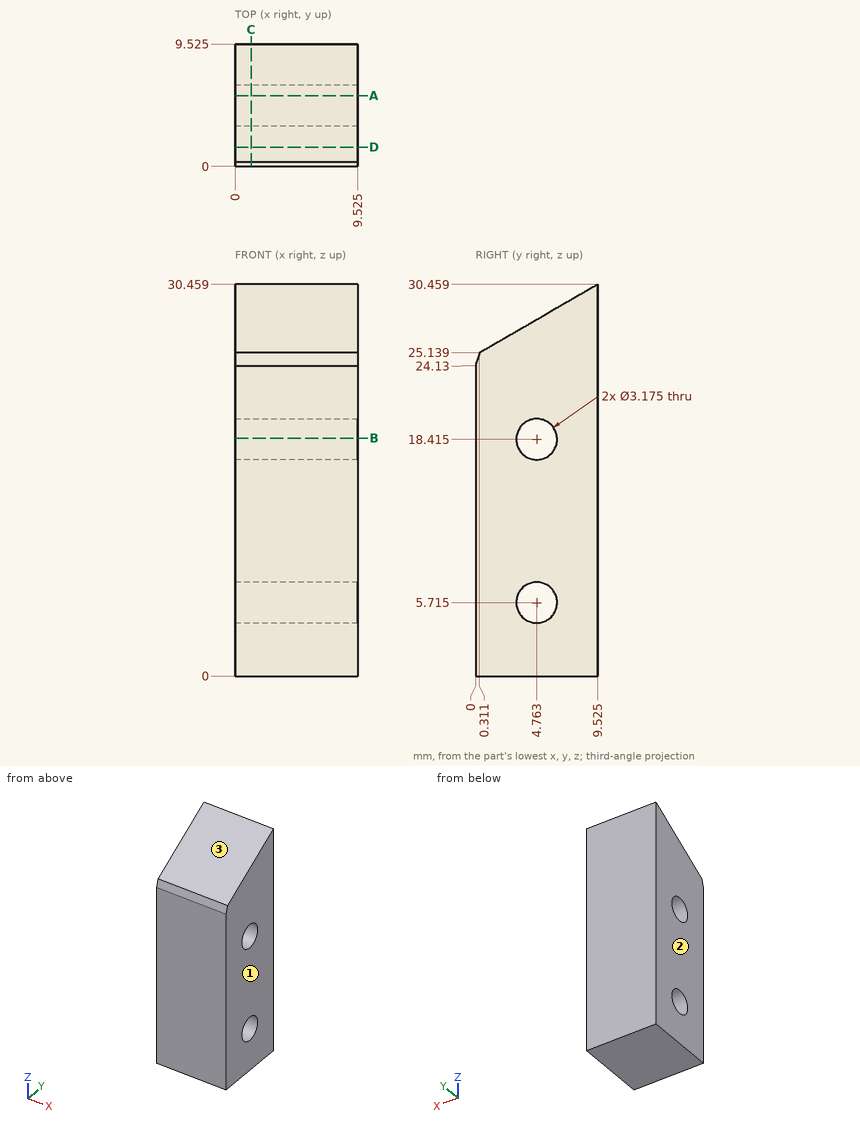
Here's the drawing with two shaded views (mm, measured from the low corner). I have some questions. Round coordinates to 2 decimals unless told otherwise and drop trailing zeros. Order: outer loops, then holes, each group sorted by start corner. A loop starts at its lowest first (then second) coordinate and runs counter-clockwise, first axis right, second up. Notation, with made-up numbers: (71, 12.5) -> (92, 12.5) arc R15 cw to (92, 37.5) -> close; hole circle Ø6 at (3.5, -25.75). An arc over 180 degrees is marked (long way). Write each question's results on one line, items separated by ' | '. Start each with the question number.
Item 1: If we section it at B-B, the plane z = 18.5: Write out the boundary of the cut face in (x, y) (1 decimal).
Item 2: If we section it at D-D, the plane y = 1.5: Write out the boundary of the cut face in (x, z) (1 decimal).
Item 3: Will these pins go through, and if not, where does the flat tip stop? pin 1 (2 mm diameter, centred on x = 5.5, z = 16, fed in from -Y); pin 2 (1 mm diameter, centred on x = 8, y = 2.5, fed in from +Z); pin 3 (4 mm diameter, centred on x = 3, y = 2, fed in from +Z); pin 4 (5 mm diameter, centred on x = 4.5, y = 3, fed in from +Z) (1 decimal).
Item 4: If we section it at A-A, the plane y = 5.5: Write out the boundary of the cut face in (x, z) (1 decimal).
Item 5: If we section it at C-C, the plane x = 1.25: Write out the boundary of the cut face in (y, z) (1 decimal), then the cut area to 3 significant figures.
Item 6: Thinking about a two-plate mould opening in X: for the marked faces 1, 2 and 3, which applies, +X half, -X half, draft (parallel to the pull), parting line (faces both ways), or undercut?
Item 7: Please list where these lines run through material, in increasing order: L1, parallel to Z at x = 7, y = 6 (1 decimal); L2, parallel to Z at x = 5, y = 3.75 (1 decimal); L3, parallel to Y at x = 1.5, z = 7 (1 decimal).
Results:
1) outline: (0, 0) -> (9.5, 0) -> (9.5, 3.2) -> (0, 3.2) -> close; (0, 6.3) -> (9.5, 6.3) -> (9.5, 9.5) -> (0, 9.5) -> close
2) outline: (0, 0) -> (9.5, 0) -> (9.5, 25.8) -> (0, 25.8) -> close
3) pin 1: stops at y = 0 | pin 2: stops at z = 26.69 | pin 3: stops at z = 27.27 | pin 4: stops at z = 28.1
4) outline: (0, 0) -> (9.5, 0) -> (9.5, 4.3) -> (0, 4.3) -> close; (0, 7.1) -> (9.5, 7.1) -> (9.5, 17) -> (0, 17) -> close; (0, 19.8) -> (9.5, 19.8) -> (9.5, 28.1) -> (0, 28.1) -> close
5) outline: (0, 0) -> (9.5, 0) -> (9.5, 30.5) -> (0.3, 25.1) -> (0, 24.1) -> close; hole circle Ø3.2 at (4.8, 5.7); hole circle Ø3.2 at (4.8, 18.4) | area: 248 mm2
6) face 1: +X half | face 2: -X half | face 3: draft
7) L1: z = 0 to 4.7, 6.7 to 17.4, 19.4 to 28.4 | L2: z = 0 to 4.5, 6.9 to 17.2, 19.6 to 27.1 | L3: y = 0 to 3.8, 5.7 to 9.5
